CAD build for the part. Positions are in the model's coordinates, mm. Face numbers are marked on the shaded views. Round coordinates to 2 decimals unless told otherwise and drop trailing zeros. Loops run counter-clockwise (first coordinate to the right, second up) from the corner with the lowest first, then second, coordinate; pieces in that order, holes last. Notation, with made-up numbers: M -38.75,35.5 L -27.75,35.5 A12 ccw -27.75,42.5 Z; hole C 50.25,11 d5. An arc over 180 degrees is marked long. One line per item, written item: value. Start each with the question number.
from build123d import *

# Parameters (mm, degrees)
F0_W     = 450
F0_H     = 450
F1_DEPTH = 950
F2_W     = 50
F2_H     = 50
F2_W_2   = 321.6566308737
F2_H_2   = 425
F3_DEPTH = 450.001
F4_W     = 378
F4_H     = 425
F5_DEPTH = 450.001
F6_W     = 378
F6_H     = 50
F6_H_2   = 302.6243293636
F7_DEPTH = 135.2537415973


with BuildPart() as f1:
    # F0 (on Top) → F1 (new body)
    with BuildSketch(Plane.XY):
        Rectangle(F0_W, F0_H)
    extrude(amount=F1_DEPTH)

    # F2 (on face) → F3 (cut, through all)
    with BuildSketch(Plane.YZ.offset(225)):
        with Locations((200, 450)):
            Rectangle(F2_W, F2_H)
        Polygon((-182.6566308737, 475), (139, 475), (189, 950), (-225, 950), (-225, 475), align=None)
        with Locations((-21.8283154368, 212.5)):
            Rectangle(F2_W_2, F2_H_2)
        with Locations((200, 212.5)):
            Rectangle(F2_W, F2_H_2)
        Polygon((175, 475), (225, 475), (225, 950), align=None)
    extrude(amount=-F3_DEPTH, mode=Mode.SUBTRACT)

    # F4 (on face) → F5 (cut, through all)
    with BuildSketch(Plane.XZ.offset(225)):
        with Locations((0, 212.5)):
            Rectangle(F4_W, F4_H)
    extrude(amount=-F5_DEPTH, mode=Mode.SUBTRACT)

    # F6 (on face) → F7 (cut, through all)
    with BuildSketch(Plane(origin=(0, 88.0246575342, -9.2657534247), x_dir=(1, 0, 0), z_dir=(0, -0.9945054529, 0.1046847845))):
        with Locations((0, 864.5656045492)):
            Rectangle(F6_W, F6_H)
        with Locations((0, 638.2534398675)):
            Rectangle(F6_W, F6_H_2)
    extrude(amount=-F7_DEPTH, mode=Mode.SUBTRACT)


solid = f1.part
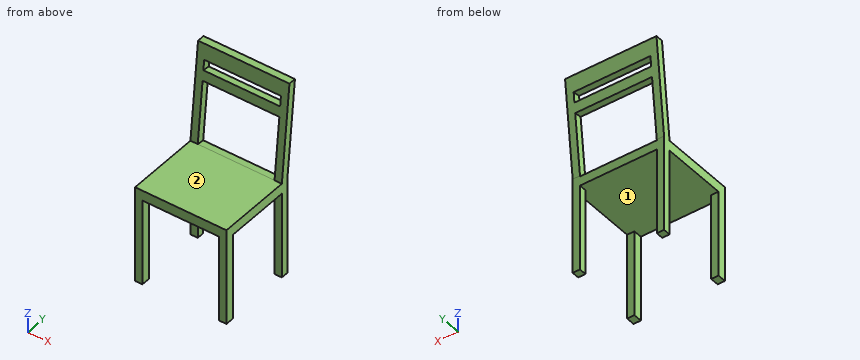
(1) Slice it at C-C, the plane z = 733. List the corners of the cut face in (x, y), and give its area (3 significant figures).
(2) Slice it at A-A, the plane x = 116. List the corners of the cut face in (y, z), and give its area (3 significant figures).
(3) Flat gauge pins, fed straight in: P1, Ø5, axis at x = -12, y = -86.5, coming from the -Z side; P2, Ø12, axis at y = 133.5, z = 299.5, coming from the +X side; P3, Ø18, axis at x = -214, z = 197.5, coming from the +Y side. Where does each tip first touch, or does it go through?
(4) Slice it at B-B, the plane z = 306. List the corners of the cut face in (x, y).
(5) Mould opens along X. For the marked faces 1 and 2 say: pulls with the +X half, pulls with the -X half, needs draft (parallel to the pull), parting line crosses it, or undercut.
(6) Slice it at D-D, the plane y = -92. List the corners of the cut face in (x, z).
(7) Probe L1, parallel to Y at x = -204, z = 242; L2, parallel to X at y = 195, z = 744; L3, parallel to Y at x = 200, z = 448. List the from-to ranges inside material, lowest first.
Check result:
1. outline: M -225,166.16 L -189,166.16 L -189,202.16 L -225,202.16 Z; M 189,166.16 L 225,166.16 L 225,202.16 L 189,202.16 Z
1. area: 2,590 mm^2
2. outline: M -225,425 L 175,425 L 175,471.21 L 139,475 L -225,475 Z; M 170.68,775.96 L 206.29,772.21 L 211.52,821.94 L 175.91,825.69 Z; M 181.15,875.41 L 216.75,871.66 L 225,950 L 189,950 Z
2. area: 24,500 mm^2
3. P1: stops at z = 425
3. P2: stops at x = 225
3. P3: stops at y = 175
4. outline: M -225,-225 L -189,-225 L -189,-182.66 L -225,-182.66 Z; M -225,139 L -189,139 L -189,175 L -225,175 Z; M 189,-225 L 225,-225 L 225,-182.66 L 189,-182.66 Z; M 189,139 L 225,139 L 225,175 L 189,175 Z
5. face 1: undercut
5. face 2: needs draft
6. outline: M -225,425 L 225,425 L 225,475 L -225,475 Z
7. L1: y = -225 to -182.66, 139 to 175
7. L2: x = -225 to -189, 189 to 225
7. L3: y = -225 to 175
